CAD build for the part. Positions are in the model's coordinates, mm. Face numbers are marked on the shaded views. Round coordinates to 2 decimals unless told otherwise and drop trailing zeros. Loops run counter-clockwise (first coordinate to the right, second up) from the corner with the lowest first, then second, coordinate; pieces in that order, holes last.
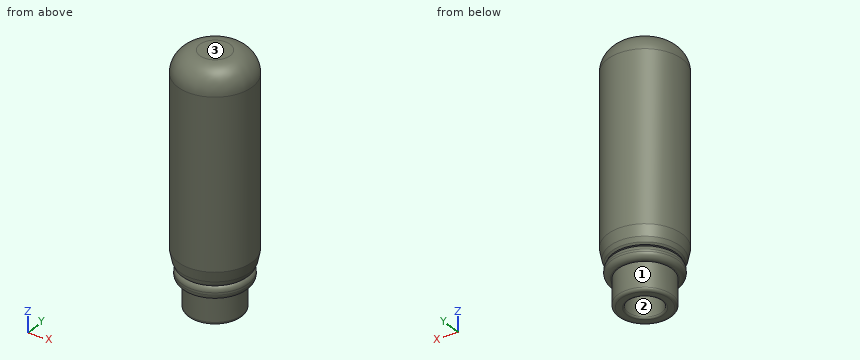
```python
from build123d import *

# Parameters (mm, degrees)
SKETCH037_R     = 4.9
PAD032_DEPTH    = 5
SKETCH038_R     = 6.1
PAD033_DEPTH    = 2.4
FILLET002_R     = 1
FILLET003_R     = 0.5
SKETCH039_R     = 6.75
PAD034_DEPTH    = 37.5
FILLET004_R     = 4
CHAMFER_SIZE    = 1
CHAMFER001_SIZE = 1
CHAMFER002_SIZE = 1
SKETCH040_R     = 3.05
POCKET008_DEPTH = 6
FILLET005_R     = 0.3


with BuildPart() as part:
    # Sketch037 → Pad032 (new body)
    with BuildSketch(Plane.XY):
        Circle(SKETCH037_R)
    extrude(amount=PAD032_DEPTH)

    # Sketch038 (on Face3 of Pad032) → Pad033 (join)
    with BuildSketch(Plane.XY.offset(5)):
        Circle(SKETCH038_R)
    extrude(amount=PAD033_DEPTH)

    # Fillet002
    fillet002_edges = [part.edges().sort_by_distance(p)[0] for p in [
        (-6.1, 0, 7.4),
        (-6.1, 0, 5),
    ]]
    fillet(fillet002_edges, radius=FILLET002_R)

    # Fillet003
    fillet003_edges = [part.edges().sort_by_distance(p)[0] for p in [
        (-4.9, 0, 0),
    ]]
    fillet(fillet003_edges, radius=FILLET003_R)

    # Sketch039 (on Face8 of Fillet003) → Pad034 (join)
    with BuildSketch(Plane.XY.offset(7.4)):
        Circle(SKETCH039_R)
    extrude(amount=PAD034_DEPTH)

    # Fillet004
    fillet004_edges = [part.edges().sort_by_distance(p)[0] for p in [
        (-6.75, 0, 44.9),
    ]]
    fillet(fillet004_edges, radius=FILLET004_R)

    # Chamfer
    chamfer_edges = [part.edges().sort_by_distance(p)[0] for p in [
        (-6.75, 0, 7.4),
    ]]
    chamfer(chamfer_edges, length=CHAMFER_SIZE)

    # Chamfer001
    chamfer001_edges = [part.edges().sort_by_distance(p)[0] for p in [
        (-6.75, 0, 8.4),
    ]]
    chamfer(chamfer001_edges, length=CHAMFER001_SIZE)

    # Chamfer002
    chamfer002_edges = [part.edges().sort_by_distance(p)[0] for p in [
        (-6.749971, 0, 9.4),
    ]]
    chamfer(chamfer002_edges, length=CHAMFER002_SIZE)

    # Sketch040 (on Face14 of Chamfer002) → Pocket008 (cut)
    with BuildSketch(Plane(origin=(0, 0, 0), x_dir=(1, 0, 0), z_dir=(0, 0, -1))):
        Circle(SKETCH040_R)
    extrude(amount=-POCKET008_DEPTH, mode=Mode.SUBTRACT)

    # Fillet005
    fillet005_edges = [part.edges().sort_by_distance(p)[0] for p in [
        (-3.05, 0, 0),
    ]]
    fillet(fillet005_edges, radius=FILLET005_R)


solid = part.part
```
Item 1: Cut at A-A, the plane z = 26.5. Give the cut face in (x, y).
Answers follow:
outline: circle Ø13.5 at (0, 0)
Item 2: Probe line 1 (Y direction, x = 0, z = 4.75); line 2 (Z direction, x = 3, y = -0.25); line 3 (Y direction, x = 3, z = 28). List the from-to ranges inside material, lowest first.
Answers follow:
line 1: y = -4.9 to -3.05, 3.05 to 4.9
line 2: z = 6 to 44.89
line 3: y = -6.05 to 6.05
Item 3: Flat gauge pins, fed straight in: P1, Ø5, axis at x = -2, y = -2.5, coming from the -Z side; P2, Ø1.8, axis at x = 1, y = -1, coming from the -Z side; P3, Ø4, axis at y = 4, z = 39.5, coming from the +X side; P4, Ø1.5, axis at x = 3, y = 4.5, coming from the +Z side. Where does each tip first touch, or does it go through?
Answers follow:
P1: stops at z = 0
P2: stops at z = 6
P3: stops at x = 6.45
P4: stops at z = 44.42
Item 4: Two-plate mould, pull along X, no slides. Class the marked faces 1, 2 and 3: released by +X, released by -X, zero draft, split by the parting line, or undercut.
Answers follow:
face 1: split by the parting line
face 2: undercut
face 3: zero draft
